Model file for the job. Use its own axes, mm. Face numbers are marked on the shaded views. Give positions to 0.01 mm unless a question says otherwise; leave off trailing zeros. Loops run counter-clockwise (first coordinate to the right, second up) from the corner with the lowest first, then second, coordinate; pieces in that order, holes last. Notation, with made-up numbers: M 13.25,-12 L 30.25,-12 A16 ccw 30.25,17 Z; hole C 40,-11 d9. An arc over 180 degrees is marked long. Answer in a Markdown table with one row per item.
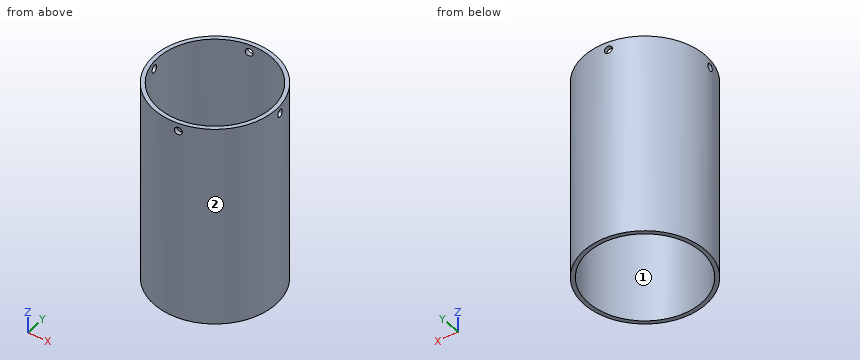
```python
from build123d import *

# Parameters (mm, degrees)
ESQUISSE1_R                  = 45
BOSS_EXTRU_1_DEPTH           = 150
ESQUISSE2_R                  = 42
ENL_V_MAT_EXTRU_1_DEPTH      = 150
D_GAGEMENT_M51_D             = 5.5
R_P_TITION_CIRCULAIRE1_COUNT = 2
R_P_TITION_CIRCULAIRE1_ANGLE = 90


with BuildPart() as part:
    # Esquisse1 → Boss.-Extru.1 (new body)
    with BuildSketch(Plane.XY):
        Circle(ESQUISSE1_R)
    extrude(amount=BOSS_EXTRU_1_DEPTH)

    # Esquisse2 → Enlèv. mat.-Extru.1 (cut)
    with BuildSketch(Plane(origin=(0, 0, 0), x_dir=(-1, 0, 0), z_dir=(0, 0, -1))):
        Circle(ESQUISSE2_R)
    extrude(amount=-ENL_V_MAT_EXTRU_1_DEPTH, mode=Mode.SUBTRACT)

    # Dégagement M51 (through all)
    with Locations(Plane(origin=(-44.649010523, -5.609443765, 144.107816194), x_dir=(0.124654306, -0.992200234, 0), z_dir=(-0.992200234, -0.124654306, 0))):
        with Locations((0, 0)):
            d_gagement_m51 = Hole(D_GAGEMENT_M51_D / 2)

    # Répétition circulaire1: Dégagement M51 ×2 about axis
    r_p_tition_circulaire1_axis = Axis((0, 0, 0), (0, 0, 1))
    for i in range(1, R_P_TITION_CIRCULAIRE1_COUNT):
        add(d_gagement_m51.rotate(r_p_tition_circulaire1_axis, i * R_P_TITION_CIRCULAIRE1_ANGLE / (R_P_TITION_CIRCULAIRE1_COUNT - 1)), mode=Mode.SUBTRACT)


solid = part.part
```
(1) Saw through at A-A, the plane y = 0. Give the cut face in (x, z), and give its area (3 significant figures).
Established:
| item | result |
|---|---|
| outline | M -45,0 L -42,0 L -42,150 L -45,150 Z; M 42,0 L 45,0 L 45,150 L 42,150 Z |
| area | 900 mm2 |
(2) Mould opens along Y. For the marked faces 1 and 2 say: pulls with the +Y half, pulls with the -Y half, needs draft (parallel to the pull), parting line crosses it, or undercut.
Established:
| item | result |
|---|---|
| face 1 | undercut |
| face 2 | parting line crosses it |
(3) Saw through at C-C, the plane z = 53.5. Give the cut face in (x, y).
Established:
| item | result |
|---|---|
| outline | C 0,0 d90; hole C 0,0 d84 |
(4) Wall check: L1, parallel to Y at x = 0, z = 72; L2, parallel to Y at x = -27, z = 134.5; L3, parallel to X at y = -24.5, z = 47.5. Give the ranges that are in metal, low to high.
Established:
| item | result |
|---|---|
| L1 | y = -45 to -42, 42 to 45 |
| L2 | y = -36 to -32.17, 32.17 to 36 |
| L3 | x = -37.75 to -34.11, 34.11 to 37.75 |
(5) Flat gauge pins, fed straight in: P1, Ø1, axis at y = -30.5, z = 23.5, coming from the +X side; P2, Ø6, axis at x = 2.5, z = 61.5, coming from the -Y side; P3, Ø1.5, axis at y = 26, z = 121, coming from the +X side. Where does each tip first touch, or does it go through?
Established:
| item | result |
|---|---|
| P1 | stops at x = 33.54 |
| P2 | stops at y = -45 |
| P3 | stops at x = 37.25 |
